```python
from build123d import *

# Parameters (mm, degrees)
SKETCH1_W           = 20
SKETCH1_H           = 20
BOSS_EXTRUDE1_DEPTH = 8
SKETCH2_R           = 3
CUT_EXTRUDE1_DEPTH  = 9
SKETCH3_R           = 1.25
CUT_EXTRUDE2_DEPTH  = 21


with BuildPart() as part:
    # Sketch1 → Boss-Extrude1 (new body)
    with BuildSketch(Plane.XY):
        with Locations((-162.646542572, -136.36630872)):
            Rectangle(SKETCH1_W, SKETCH1_H)
    extrude(amount=BOSS_EXTRUDE1_DEPTH)

    # Sketch2 → Cut-Extrude1 (cut, through all)
    with BuildSketch(Plane.XY.offset(8)):
        with Locations((-162.646542572, -136.36630872)):
            Circle(SKETCH2_R)
    extrude(amount=-CUT_EXTRUDE1_DEPTH, mode=Mode.SUBTRACT)

    # Sketch3 → Cut-Extrude2 (cut, through all)
    with BuildSketch(Plane(origin=(-152.646542572, 0, 0), x_dir=(0, 0, -1), z_dir=(1, 0, 0))):
        with Locations((-4, -136.36630872)):
            Circle(SKETCH3_R)
    extrude(amount=-CUT_EXTRUDE2_DEPTH, mode=Mode.SUBTRACT)


solid = part.part
```
Work out the finished part from the listing and answer in its coordinate system (mm). Give positions to 0.01 mm unless a question says otherwise; leave off trailing zeros. Loops run counter-clockwise (first coordinate to the right, second up) from the corner with the lowest first, then second, coordinate; pieces in that order, holes last. Notation, with made-up numbers: (55, 82) -> (94, 82) arc R27 ccw to (94, 120) -> close; hole circle Ø11 at (-24, -21). An arc over 180 degrees is marked (long way). One line per question, with ' | ' between items. Start each with the question number.
1) Section D-D, the plane z = 6.25 is taken. Determine the outline of the cut face in (x, y), then the cut area to 3 significant figures.
2) Section A-A, the plane z = 4 is taken. Determine the outline of the cut face in (x, y).
3) Section B-B, the plane y = -138.75 is taken. Determine the outline of the cut face in (x, z) (3 decimals), then the cut area to 3 significant figures.
4) Section C-C, the plane x = -169.5 is taken. Determine the outline of the cut face in (y, z), then the cut area to 3 significant figures.
5) This flat-tipped pin is pushed along its axis until it touches: pin 1 (10 mm diameter, centred on x = -168, y = -140, fed in from -Z). Where does it stop, or does it pass through?
6) Determine the mould class of faces 1 (the face through (-161.262, -139.028, 4.056)), 2 (the face through (-163, -146.366, 4)), 3 (the face through (-172.647, -137, 2)) for opening direction X: +X half, -X half, draft (parallel to the pull), parting line (faces both ways), or undercut.
7) Straight lines are drawn through the part: L1, parallel to Y at x = -162.75, z = 4.75; L2, parallel to X at y = -139, z = 6.75; L3, parallel to X at y = -134.5, z = 2.75. For each, find the intervals that lie inside material, in ascending order.
Resolved:
1) outline: (-172.65, -146.37) -> (-152.65, -146.37) -> (-152.65, -126.37) -> (-172.65, -126.37) -> close; hole circle Ø6 at (-162.65, -136.37) | area: 372 mm2
2) outline: (-172.65, -146.37) -> (-152.65, -146.37) -> (-152.65, -137.62) -> (-159.92, -137.62) arc R3 cw to (-165.37, -137.62) -> (-172.65, -137.62) -> close; (-172.65, -135.12) -> (-165.37, -135.12) arc R3 cw to (-159.92, -135.12) -> (-152.65, -135.12) -> (-152.65, -126.37) -> (-172.65, -126.37) -> close
3) outline: (-172.647, 0) -> (-164.468, 0) -> (-164.468, 8) -> (-172.647, 8) -> close; (-160.825, 0) -> (-152.647, 0) -> (-152.647, 8) -> (-160.825, 8) -> close | area: 131 mm2
4) outline: (-146.37, 0) -> (-126.37, 0) -> (-126.37, 8) -> (-146.37, 8) -> close; hole circle Ø2.5 at (-136.37, 4) | area: 155 mm2
5) pin 1: z = 0
6) face 1: undercut | face 2: draft | face 3: -X half
7) L1: -146.37 to -139.36, -133.37 to -126.37 | L2: -172.65 to -164.08, -161.21 to -152.65 | L3: -172.65 to -165, -160.3 to -152.65
